Source: CAD feature listing. Evaluate the final solid. Frame: model axes, mm. A direction names the side the tool comes from. Round coordinates to 2 decimals unless told otherwise and drop trailing zeros. Loops run counter-clockwise (first coordinate to the right, second up) from the corner with the lowest first, then second, coordinate; pieces in that order, holes last.
(1) Material intervals for probe 1 along Y at (x, z) = (-46.5, 23.75); probe 2 along Z at (x, y) = (-12, 5.5); probe 3 along Z at (x, y) = (-8, 2.75), sorted ascending.
(2) Mould query, pull axis X, two halves, no side actions, for faces 4 (the flat face through (-28, 4, -5)), 5 (the flat face through (-23, 4.874, 15)). Classes: pulls with the +X half, pulls with the -X half, needs draft (parallel to the pull), parting line crosses it, or undercut.
(3) Section A-A, the plane y = 8. Return the cut outline in (x, z).
(4) Section B-B, the plane z = 14.25. Count the separate pieces of the cut face and the enclosed holes in it, plus the area to 3 significant figures.
(5) Set-up query: faces 1 (the flat face through (-15.05, 3.92, 7.96)), 2 (the flat face through (-7, 5.374, 12)), 3 (the flat face through (-29.93, 3.19, -0.01)). Return all of +Z, -Z, +X, -X, +Y, -Y with unobstructed straight access to the full face (end or side cutting, diameter ignored); none if empty.
(6) First-contact query: pin 1 Ø3 at (x, y) = (-45, 6) entering from -Z; pin 2 Ø1.2 at (x, z) = (-48.5, 15) entering from +Y; pin 3 Ø1.5 at (x, y) = (-27, 4) entering from +Z. Flat tips, straight axial feed; report the tip coordinate or a pass-through.
(7) Section D-D, the plane z = 5.5. Return the cut outline in (x, y).
(8) Section C-C, the plane x = -15. Return the cut outline in (y, z).
```python
from build123d import *

# Parameters (mm, degrees)
SKETCH_1_R           = 3.1
SKETCH_1_R_2         = 1.6
EXTRUDE_1_DEPTH      = 25
EXTRUDE_2_DEPTH      = 2.945
CUT_EXTRUDE_1_DEPTH  = 56.64644355
CUT_EXTRUDE_START    = -1.5
CUT_EXTRUDE_4_DEPTH  = 1.5
SKETCH_6_R           = 0.8
CUT_EXTRUDE_5_DEPTH  = 56.64644355
CUT_EXTRUDE_6_DEPTH  = 56.64644355
SKETCH_9_W           = 14
SKETCH_9_H           = 3.255
CUT_EXTRUDE_9_DEPTH  = 46.904396246
SKETCH_10_R          = 1.4
CUT_EXTRUDE_11_DEPTH = 0.5
CUT_EXTRUDE_12_DEPTH = 0.4


with BuildPart() as part:
    # 草图1 → 凸台-拉伸1 (new body)
    # profile 1 of 3: a face of its own
    with BuildSketch(Plane.XY):
        with Locations((-46.507778168, 5.529205914)):
            Circle(SKETCH_1_R)
        with Locations((-46.507778168, 5.529205914)):
            Circle(SKETCH_1_R_2, mode=Mode.SUBTRACT)
    # profile 2 of 3: a face of its own
    with BuildSketch(Plane.XY):
        with BuildLine():
            ThreePointArc((-43.411655593, 5.374205914), (-44.371250611, 3.283042519), (-46.507778168, 2.429205914))
            Line((-46.507778168, 2.429205914), (-8.987778168, 2.429205914))
            ThreePointArc((-8.987778168, 2.429205914), (-11.124305724, 3.283042519), (-12.083900743, 5.374205914))
            Line((-12.083900743, 5.374205914), (-43.411655593, 5.374205914))
        make_face()
    # profile 3 of 3: a face of its own
    with BuildSketch(Plane.XY):
        with Locations((-8.987778168, 5.529205914)):
            Circle(SKETCH_1_R)
        with Locations((-8.987778168, 5.529205914)):
            Circle(SKETCH_1_R_2, mode=Mode.SUBTRACT)
    extrude(amount=EXTRUDE_1_DEPTH)

    # 草图2 → 凸台-拉伸2 (add)
    with BuildSketch(Plane(origin=(0, 5.374205914, 0), x_dir=(1, 0, 0), z_dir=(0, 1, 0))):
        Polygon((-19.247778168, 0), (-24.247778168, 5), (-31.247778168, 5), (-36.247778168, 0), align=None)
    extrude(amount=-EXTRUDE_2_DEPTH)

    # 草图3 → 切除-拉伸1 (cut, through all)
    with BuildSketch(Plane(origin=(0, 5.374205914, 0), x_dir=(1, 0, 0), z_dir=(0, 1, 0))):
        with BuildLine():
            Line((-28.147778168, 0), (-27.347778168, 0))
            ThreePointArc((-27.347778168, 0), (-26.347778168, -1), (-27.347778168, -2))
            Line((-27.347778168, -2), (-28.147778168, -2))
            ThreePointArc((-28.147778168, -2), (-29.147778168, -1), (-28.147778168, 0))
        make_face()
    extrude(amount=-CUT_EXTRUDE_1_DEPTH, mode=Mode.SUBTRACT)

    # 草图5 → 切除-拉伸4 (cut)
    # profile 1 of 3: a face of its own
    with BuildSketch(Plane(origin=(0, 2.429205914, 0), x_dir=(-1, 0, 0), z_dir=(0, -1, 0)).offset(CUT_EXTRUDE_START)):
        Polygon((25.780642064, -1), (26.964210116, 1.05), (26.164210116, 1.05), (24.980642064, -1), (26.164210116, -3.05), (26.964210116, -3.05), align=None)
    # profile 2 of 3: a face of its own
    with BuildSketch(Plane(origin=(0, 2.429205914, 0), x_dir=(-1, 0, 0), z_dir=(0, -1, 0)).offset(CUT_EXTRUDE_START)):
        Polygon((28.53134622, -3.05), (29.714914272, -1), (28.53134622, 1.05), (26.964210116, 1.05), (25.780642064, -1), (26.964210116, -3.05), align=None)
        with BuildLine():
            ThreePointArc((27.347778168, -2), (26.347778168, -1), (27.347778168, 0))
            Line((27.347778168, 0), (28.147778168, 0))
            ThreePointArc((28.147778168, 0), (29.147778168, -1), (28.147778168, -2))
            Line((28.147778168, -2), (27.347778168, -2))
        make_face(mode=Mode.SUBTRACT)
    # profile 3 of 3: a face of its own
    with BuildSketch(Plane(origin=(0, 2.429205914, 0), x_dir=(-1, 0, 0), z_dir=(0, -1, 0)).offset(CUT_EXTRUDE_START)):
        Polygon((28.53134622, 1.05), (29.714914272, -1), (28.53134622, -3.05), (29.33134622, -3.05), (30.514914272, -1), (29.33134622, 1.05), align=None)
    extrude(amount=CUT_EXTRUDE_4_DEPTH, mode=Mode.SUBTRACT)

    # 草图6 → 切除-拉伸5 (cut, through all)
    with BuildSketch(Plane(origin=(0, 5.374205914, 0), x_dir=(1, 0, 0), z_dir=(0, 1, 0))):
        with Locations(Location((-32.747778168, -14, 0), (0, 0, 270))):
            Circle(SKETCH_6_R)
        with Locations(Location((-22.747778168, -14, 0), (0, 0, 270))):
            Circle(SKETCH_6_R)
    extrude(amount=-CUT_EXTRUDE_5_DEPTH, mode=Mode.SUBTRACT)

    # 草图7 → 切除-拉伸6 (cut, through all)
    with BuildSketch(Plane(origin=(0, 5.374205914, 0), x_dir=(1, 0, 0), z_dir=(0, 1, 0))):
        Polygon((-35.407778168, -17), (-43.407778168, -25), (-12.083900743, -25), (-20.083900743, -17), align=None)
        Polygon((-37.407778168, -13), (-37.407778168, -11), (-43.407778168, -5), (-43.407778168, -19), align=None)
        Polygon((-12.087778168, -5), (-18.087778168, -11), (-18.087778168, -13), (-12.087778168, -19), align=None)
    extrude(amount=-CUT_EXTRUDE_6_DEPTH, mode=Mode.SUBTRACT)

    # 草图9 → 切除-拉伸9 (cut, through all)
    with BuildSketch(Plane.ZY.offset(12.087778168)):
        with Locations((12, 7.001705914)):
            Rectangle(SKETCH_9_W, SKETCH_9_H)
    cut_extrude_9 = extrude(amount=-CUT_EXTRUDE_9_DEPTH, mode=Mode.SUBTRACT)

    # 镜向1: 切除-拉伸9 across plane
    add(cut_extrude_9.mirror(Plane(origin=(-27.747778168, 0, 0), x_dir=(0, 0, 1), z_dir=(1, 0, 0))), mode=Mode.SUBTRACT)

    # 草图10 → 切除-拉伸11 (cut)
    with BuildSketch(Plane(origin=(0, 5.374205914, 0), x_dir=(1, 0, 0), z_dir=(0, 1, 0))):
        with Locations(Location((-22.747778168, -14, 0), (0, 0, 270))):
            Circle(SKETCH_10_R)
        with Locations(Location((-32.747778168, -14, 0), (0, 0, 270))):
            Circle(SKETCH_10_R)
    extrude(amount=-CUT_EXTRUDE_11_DEPTH, mode=Mode.SUBTRACT)

    # 草图11 → 切除-拉伸12 (cut)
    with BuildSketch(Plane(origin=(0, 5.374205914, 0), x_dir=(1, 0, 0), z_dir=(0, 1, 0))):
        with BuildLine():
            Line((-27.247778168, -4.65), (-28.247778168, -4.65))
            ThreePointArc((-28.247778168, -4.65), (-31.897778168, -1), (-28.247778168, 2.65))
            Line((-28.247778168, 2.65), (-27.247778168, 2.65))
            ThreePointArc((-27.247778168, 2.65), (-23.597778168, -1), (-27.247778168, -4.65))
        make_face()
    extrude(amount=-CUT_EXTRUDE_12_DEPTH, mode=Mode.SUBTRACT)


solid = part.part
```
Output values:
1. probe 1: y = 2.43 to 3.93, 7.13 to 8.63
1. probe 2: z = 0 to 5, 19 to 25
1. probe 3: z = 0 to 25
2. face 4: needs draft
2. face 5: undercut
3. outline: (-48.38, 0) - (-44.64, 0) - (-44.64, 5) - (-48.38, 5) - close; (-48.38, 19) - (-44.64, 19) - (-44.64, 25) - (-48.38, 25) - close; (-10.86, 0) - (-7.12, 0) - (-7.12, 5) - (-10.86, 5) - close; (-10.86, 19) - (-7.12, 19) - (-7.12, 25) - (-10.86, 25) - close
4. separate pieces: 5
4. enclosed holes: 0
4. area: 79.4 mm2
5. face 1: +Y, -Y
5. face 2: +X, -X, +Y
5. face 3: -Y
6. pin 1: stops at z = 0
6. pin 2: stops at y = 5.37
6. pin 3: stops at z = 17
7. outline: (-49.6, 5.37) arc R3.1 ccw to (-46.51, 2.43) - (-43.41, 2.43) - (-43.41, 5.37) - (-44.92, 5.37) arc R1.6 cw to (-48.1, 5.37) - close; (-42.91, 2.43) - (-12.59, 2.43) - (-12.59, 5.37) - (-42.91, 5.37) - close; (-12.09, 2.43) - (-8.99, 2.43) arc R3.1 ccw to (-5.89, 5.37) - (-7.4, 5.37) arc R1.6 cw to (-10.58, 5.37) - (-12.09, 5.37) - close
8. outline: (2.43, 0) - (5.37, 0) - (5.37, 7.91) - (2.43, 7.91) - close; (2.43, 16.09) - (5.37, 16.09) - (5.37, 22.08) - (2.43, 22.08) - close
